from build123d import *

# Parameters (mm, degrees)
SKETCH1_R           = 76.1746
SKETCH1_R_2         = 73.66
BOSS_EXTRUDE1_DEPTH = 330.2
SKETCH23_R          = 1.0922
SHEAR_SCRREWS_DEPTH = 108.72715257
CIRPATTERN1_COUNT   = 4


with BuildPart() as part:
    # Sketch1 → Boss-Extrude1 (new body)
    with BuildSketch(Plane(origin=(0, 0, 0), x_dir=(1, 0, 0), z_dir=(0, 1, 0))):
        Circle(SKETCH1_R)
        Circle(SKETCH1_R_2, mode=Mode.SUBTRACT)
    extrude(amount=BOSS_EXTRUDE1_DEPTH)

    # Sketch17 → 1/2 Clearance Hole5 (revolve, cut)
    with BuildSketch(Plane(origin=(0, 288.925, 0), x_dir=(0, -1, 0), z_dir=(1, 0, 0))):
        Polygon((0, 0), (0, 80.134507437), (6.54812, 76.2), (6.54812, 0), align=None)
    revolve(axis=Axis((0, 288.925, 6.35), (0, 0, -1)), mode=Mode.SUBTRACT)

    # Sketch21 → 1/2 Clearance Hole7 (revolve, cut)
    with BuildSketch(Plane(origin=(0, 41.275, 0), x_dir=(0, -1, 0), z_dir=(1, 0, 0))):
        Polygon((0, 0), (0, 80.134507437), (6.54812, 76.2), (6.54812, 0), align=None)
    revolve(axis=Axis((0, 41.275, 6.35), (0, 0, -1)), mode=Mode.SUBTRACT)

    # Sketch23 → Shear Scrrews (cut, through all)
    with BuildSketch(Plane(origin=(0, 0, 0), x_dir=(0.707106781, 0, 0.707106781), z_dir=(-0.707106781, 0, 0.707106781))):
        with Locations((0, 292.1)):
            Circle(SKETCH23_R)
        with Locations((0, 38.1)):
            Circle(SKETCH23_R)
    shear_scrrews = extrude(amount=-SHEAR_SCRREWS_DEPTH, mode=Mode.SUBTRACT)

    # CirPattern1: Shear Scrrews ×4 about axis
    cirpattern1_axis = Axis((0, 330.2, 0), (0, -1, 0))
    for i in range(1, CIRPATTERN1_COUNT):
        add(shear_scrrews.rotate(cirpattern1_axis, i * 360 / CIRPATTERN1_COUNT), mode=Mode.SUBTRACT)


solid = part.part
The listing builds one solid part. Answer for the finished solid, in the listing's coordinates (mm). A direction names the side the tool comes from. Coordinates: 2 decimals unless noted, no trailing zeros. Loops run counter-clockwise (first coordinate to the right, second up) from the corner with the lowest first, then second, coordinate; pieces in that order, holes last. Notation, with made-up numbers: (47.25, -28) -> (80.25, -28) arc R21 ccw to (80.25, -14) -> close; hole circle Ø3 at (32.25, -23). An arc over 180 degrees is marked (long way). Answer in a Markdown table with one row per item. Add a question column.
1. Consider line 1 (Y direction, x = 0, z = -74.1); line 2 (Z direction, x = 0, y = 232.5); line 3 (Z direction, x = -3.5, y = 259). Determine where each line is inside the solid, lowest interval first. Write a range as [from, to].
2. The part is cut by section B-B, the plane x = 21. Write down the section's boundary in (y, z).
3. Determine the mould class of faces 3 (the flat face through (-39.9, 0, -62.4)), 4 (the flat face through (-39.9, 330.2, -62.4)), 5 (the cylindrical face through (-1.97, 282.68, -74.75)) for opening direction Y: +Y half, -Y half, draft (parallel to the pull), parting line (faces both ways), or undercut.
4. Flat-ended cylindrical pins translate along their axes: P1, Ø3, axis at x = 27, y = 260.5, coming from the -Z side; P2, Ø10, axis at x = 40.5, y = 174, coming from the -Z side; P3, Ø2, axis at x = -49.5, y = 114.5, coming from the -Z side. Find the tip coordinate at first contact, or state that the pin passes through.
5. The part is cut by section A-A, the plane z = 0. Write down the section's boundary in (x, y), then the cut area to 3 significant figures.
6. The part is cut by section D-D, the plane y = 198.5. Write down the section's boundary in (x, z), then the cut area to 3 significant figures.
7. The part is cut by section C-C, the plane x = 0. Write down the section's boundary in (y, z), then the cut area to 3 significant figures.
8. For faces 1 (the cylindrical face through (-1.97, 35.03, -74.75)), 2 (the cylindrical face through (-16.513, 162.789, 74.363)), determine the directions among +Z, -Z, +X, -X, +Y, -Y from which every point of the face is accessible in a straight line to the end or side of a thin tool.
Answer below:
| question | item | result |
|---|---|---|
| 1 | line 1 | [0, 34.73], [47.82, 282.38], [295.47, 330.2] |
| 1 | line 2 | [-76.17, -73.66], [73.66, 76.17] |
| 1 | line 3 | [-76.09, -73.58], [73.58, 76.09] |
| 2 | outline | (0, -73.22) -> (330.2, -73.22) -> (330.2, -70.6) -> (0, -70.6) -> close; (0, 70.6) -> (330.2, 70.6) -> (330.2, 73.22) -> (0, 73.22) -> close |
| 3 | face 3 | -Y half |
| 3 | face 4 | +Y half |
| 3 | face 5 | undercut |
| 4 | P1 | z = -71.78 |
| 4 | P2 | z = -67.4 |
| 4 | P3 | z = -58.74 |
| 5 | outline | (-76.17, 0) -> (-73.66, 0) -> (-73.66, 330.2) -> (-76.17, 330.2) -> close; (73.66, 0) -> (76.17, 0) -> (76.17, 330.2) -> (73.66, 330.2) -> close |
| 5 | area | 1,660 mm2 |
| 6 | outline | circle Ø152.35 at (0, 0); hole circle Ø147.32 at (0, 0) |
| 6 | area | 1,180 mm2 |
| 7 | outline | (0, -76.17) -> (34.73, -76.17) -> (34.73, -73.66) -> (0, -73.66) -> close; (0, 73.66) -> (330.2, 73.66) -> (330.2, 76.17) -> (0, 76.17) -> close; (47.82, -76.17) -> (282.38, -76.17) -> (282.38, -73.66) -> (47.82, -73.66) -> close; (295.47, -76.17) -> (330.2, -76.17) -> (330.2, -73.66) -> (295.47, -73.66) -> close |
| 7 | area | 1,590 mm2 |
| 8 | face 1 | -Z |
| 8 | face 2 | +Y, -Y |
